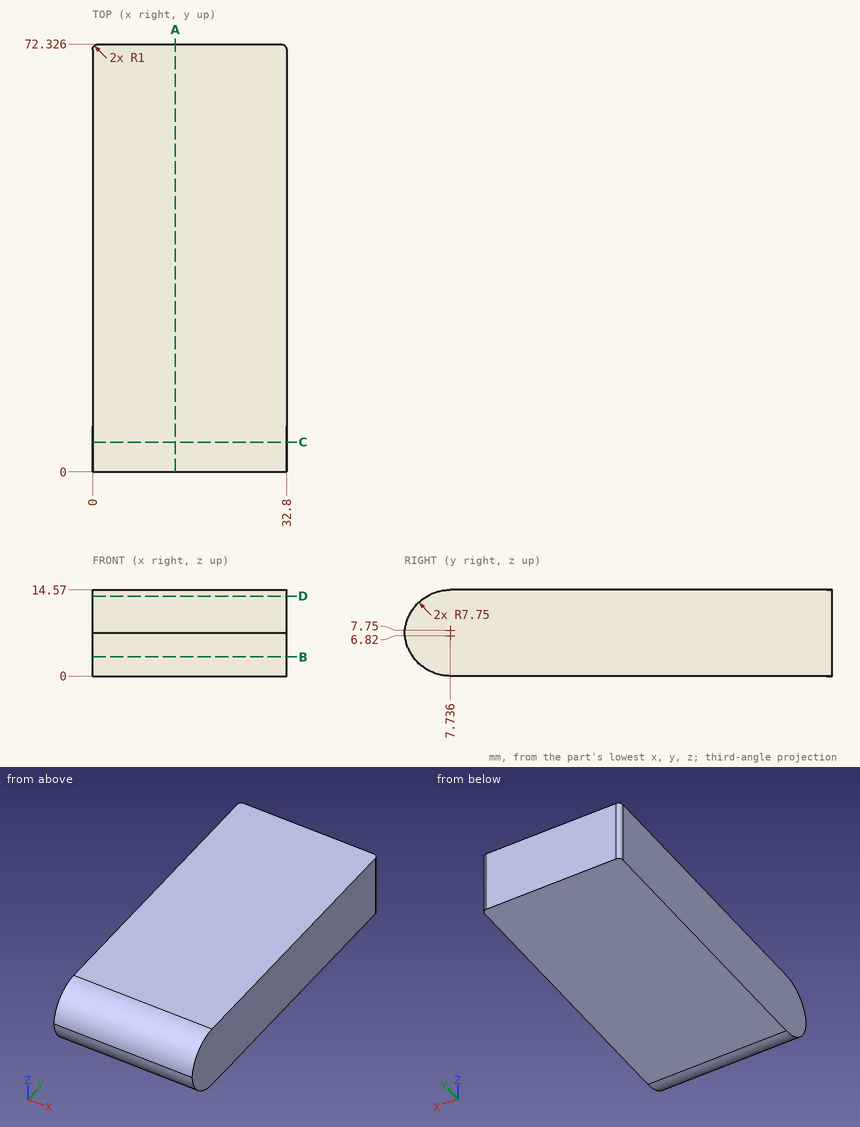
Geometry check sheet. Reference: drawing and pictorial views, mm from the part's lowest x, y, z. Give positions to 0.01 mm unless a question says otherwise; leave off trailing zeros. Write each loop counter-clockwise with the first axis right and the second up, starting at its lowest first coordinate (ties: lowest second). Pieces come first, ordered by that corner, then holes. Notation, with made-up numbers: (69, -39.75) -> (100, -39.75) arc R29 ccw to (100, -1.75) -> close; hole circle Ø8 at (36, 42.25). An arc over 180 degrees is marked (long way). One line per question, with ' | ' between items.
Item 1: Sectioned sample at A-A, the plane x = 14. Record the boundary of the cut face in (y, z) (3 decimals), plus the area to 3 significant figures.
Determined:
outline: (0, 7.285) arc R7.75 ccw to (7.736, 0) -> (72.326, 0) -> (72.326, 14.57) -> (7.736, 14.57) arc R7.75 ccw to start | area: 1,030 mm^2
Item 2: Scan lines: line 1 along Y through (x, z) = (31.5, 13.25); line 2 along Y through (x, z) = (6.5, 2); line 3 along Z through (x, y) = (6.5, 7) (3 decimals). Record each from-to range of solid material in increasing order.
Determined:
line 1: 3.41 to 72.33 | line 2: 2.54 to 72.33 | line 3: 0.035 to 14.535
Item 3: Sectioned sample at D-D, the plane z = 13.5. Record the boundary of the cut face in (x, y).
Determined:
outline: (0, 3.81) -> (32.8, 3.81) -> (32.8, 71.33) arc R1 ccw to (31.8, 72.33) -> (1, 72.33) arc R1 ccw to (0, 71.33) -> close
Item 4: Depth check by flat-ended pin: pin 1 (8 mm diameter, centred on x = 16, z = 12.5, fed in from -Y). Enter the tip coordinate at first touch or a pass-through.
Determined:
pin 1: y = 0.17
Item 5: Sectioned sample at B-B, the plane z = 3.25. Record the boundary of the cut face in (x, y), plus the area to 3 significant figures.
Determined:
outline: (0, 1.43) -> (32.8, 1.43) -> (32.8, 71.33) arc R1 ccw to (31.8, 72.33) -> (1, 72.33) arc R1 ccw to (0, 71.33) -> close | area: 2,330 mm^2
Item 6: Sectioned sample at C-C, the plane y = 5. Record the boundary of the cut face in (x, z), plus the area to 3 significant figures.
Determined:
outline: (0, 0.5) -> (32.8, 0.5) -> (32.8, 14.07) -> (0, 14.07) -> close | area: 445 mm^2
